Can you work these out from the model? Positions are in its coordinate system, mm. Face numbers are marked on the shaded views. A direction names the side the tool comes from. Coordinates: 2 decimals unless noted, no trailing zeros. Order: outer loops, then holes, each group sorted by start corner. A loop starts at its lowest first (then second) coordinate and runs counter-clockwise, first axis right, second up. Notation, with made-up numbers: (19, -4.75) -> (59, -4.75) arc R8 cw to (59, 0.25) -> close; hole circle Ø2 at (1, 72). An arc over 180 degrees is marked (long way). Return JSON: item names as keys, results as strings. Group by question number.
1) Thinking about a two-plate mould opening in X: for the marked faces 1, 2 and 3, which applies, +X half, -X half, draft (parallel to the pull), parting line (faces both ways), or undercut?
2) For pin 1 (5.5 mm diameter, centred on x = 51.08, y = 51.08, fed in from +Z); pin 2 (1.5 mm diameter, centred on x = 43, y = 14.5, fed in from +Z) (3 decimals), each with a flat end and sliding along its axis, tell me the tip position at first contact or that it passes through.
3) For the marked faces 4 and 5, which set-ups out of +Z, -Z, +X, -X, +Y, -Y let a thin tool reach every point of the face, with its end or its side?
4) If we section it at A-A, the plane x = 19.5: Please give me the cut outline in (y, z) (3 decimals).
5) If we section it at D-D, the plane y = 19: Please give me the cut outline in (x, z) (3 decimals).
6) If I drill on probe 1 along X at (y, z) = (51, 5.75); probe 2 along X at (y, z) = (53, 9.5); probe 3 along X at (y, z) = (26, 8.25), over which ranges is the centre line in solid material (lowest first)? Write a range as from..to.
7) If we section it at C-C, the plane x = 8: Please give me the cut outline in (y, z) (3 decimals).
8) If we section it at B-B, the plane z = 4.25: Please give me the cut outline in (x, y) (3 decimals), then the cut area to 3 significant figures.
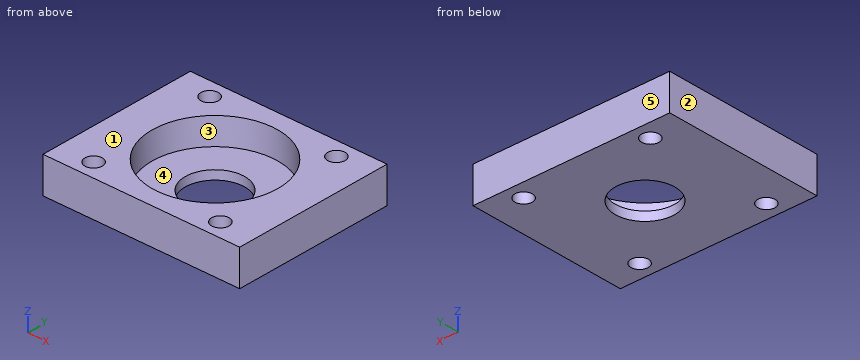
Autodesk Inventor part; units mm, degrees
ref_plane "YZ Plane" through (0, 0, 0) normal (1, 0, 0) x (0, 1, 0)
ref_plane "XZ Plane" through (0, 0, 0) normal (0, 1, 0) x (-1, 0, 0)
ref_plane "XY Plane" through (0, 0, 0) normal (0, 0, 1) x (1, 0, 0)
sketch "Sketch1" plane through (0, 0, 0) normal (0, 0, 1) x (1, 0, 0)
  line L0 (0, 0) -> (57.15, 0)
  line L1 (57.15, 0) -> (57.15, 57.15)
  line L2 (57.15, 57.15) -> (0, 57.15)
  line L3 (0, 57.15) -> (0, 0)
  line L4 (0, 57.15) -> (57.15, 0) construction
  circle A0 centre (28.575, 28.575) radius 31.825 construction
  line L5 (0, 0) -> (57.15, 57.15) construction
  circle A1 centre (6.0713, 51.0787) radius 3.1
  circle A2 centre (6.0713, 6.0713) radius 3.1
  circle A3 centre (51.0787, 6.0713) radius 3.1
  circle A4 centre (51.0787, 51.0787) radius 3.1
  circle A5 centre (28.575, 28.575) radius 11.1125
  dimension "d2" = 63.65
  dimension "d0" = 57.15
  dimension "d1" = 57.15
  dimension "d3" = 6.2
  dimension "d6" = 360
  dimension "d10" = 22.225
extrude "Extrusion1" add sketch "Sketch1" along normal blind 12.7 contours L3 L2 L1 L0 | A5
sketch "Sketch2" plane through (0, 0, 12.7) normal (0, 0, 1) x (1, 0, 0)
  circle A0 centre (28.575, 28.575) radius 10.5
  line L0 (57.15, 57.15) -> (0, 57.15)
  line L1 (57.15, 0) -> (57.15, 57.15)
  point P0 (0, 0)
  dimension "d11" = 21
  dimension "d12" = 28.575
  dimension "d13" = 28.575
extrude "Extrusion2" cut sketch "Sketch2" against normal blind 25.4
sketch "Sketch3" plane through (0, 0, 12.7) normal (0, 0, 1) x (1, 0, 0)
  circle A0 centre (28.575, 28.575) radius 10.5
  circle A1 centre (28.575, 28.575) radius 22.225
  point P0 (0, 0)
  dimension "d16" = 44.45
extrude "Extrusion3" cut sketch "Sketch3" against normal blind 9.525
sketch "Sketch4" plane through (0, 0, 12.7) normal (0, 0, 1) x (1, 0, 0)
  line L0 (0, 57.15) -> (0, 0)
  line L1 (0, 57.15) -> (-6.35, 57.15)
  line L2 (-6.35, 57.15) -> (-6.35, 0)
  line L3 (-6.35, 0) -> (0, 0)
  line L4 (0, 0) -> (0, 57.15)
  line L5 (57.15, 0) -> (57.15, 57.15)
  line L6 (57.15, 57.15) -> (63.5, 57.15)
  line L7 (63.5, 57.15) -> (63.5, 0)
  line L8 (63.5, 0) -> (57.15, 0)
  line L9 (57.15, 0) -> (57.15, 57.15)
  dimension "d19" = 6.35
  dimension "d20" = 6.35
extrude "Extrusion4" add sketch "Sketch4" against normal up to surface (12.7 mm away)
sketch "Sketch5" plane through (0, 0, 12.7) normal (0, 0, 1) x (1, 0, 0)
  circle A0 centre (28.575, 28.575) radius 10.5
  circle A1 centre (51.0787, 6.0713) radius 3.1
  circle A2 centre (28.575, 28.575) radius 31.825
  point P0 (0, 0)
properties part number "polycarb_front" material "Polycarbonate, Smoke"
Result sheet:
{
 "1": {"face 1": "draft", "face 2": "-X half", "face 3": "undercut"},
 "2": {"pin 1": "passes through", "pin 2": "stops at z = 3.175"},
 "3": {"face 4": "+Z", "face 5": "+Z, -Z, +X, -X, +Y"},
 "4": {"outline": "(0, 0) -> (23.293, 0) -> (23.293, 3.175) -> (8.287, 3.175) -> (8.287, 12.7) -> (0, 12.7) -> close; (33.857, 0) -> (57.15, 0) -> (57.15, 12.7) -> (48.863, 12.7) -> (48.863, 3.175) -> (33.857, 3.175) -> close"},
 "5": {"outline": "(-6.35, 0) -> (24.266, 0) -> (24.266, 3.175) -> (8.518, 3.175) -> (8.518, 12.7) -> (-6.35, 12.7) -> close; (32.884, 0) -> (63.5, 0) -> (63.5, 12.7) -> (48.632, 12.7) -> (48.632, 3.175) -> (32.884, 3.175) -> close"},
 "6": {"probe 1": "x = -6.35..2.97, 9.17..47.98, 54.18..63.5", "probe 2": "x = -6.35..3.64, 8.5..48.65, 53.51..63.5", "probe 3": "x = -6.35..6.5, 50.65..63.5"},
 "7": {"outline": "(0, 0) -> (3.644, 0) -> (3.644, 12.7) -> (0, 12.7) -> close; (8.498, 0) -> (48.652, 0) -> (48.652, 12.7) -> (36.979, 12.7) -> (36.979, 3.175) -> (20.171, 3.175) -> (20.171, 12.7) -> (8.498, 12.7) -> close; (53.506, 0) -> (57.15, 0) -> (57.15, 12.7) -> (53.506, 12.7) -> close"},
 "8": {"outline": "(-6.35, 0) -> (63.5, 0) -> (63.5, 57.15) -> (-6.35, 57.15) -> close; hole circle Ø6.2 at (6.071, 6.071); hole circle Ø6.2 at (6.071, 51.079); hole circle Ø44.45 at (28.575, 28.575); hole circle Ø6.2 at (51.079, 6.071); hole circle Ø6.2 at (51.079, 51.079)", "area": "2,320 mm2"}
}
